Here's how the part is built. I have some questions about the finished solid (model axes, mm). Round coordinates to 2 decimals unless told otherwise and drop trailing zeros. Write each loop counter-clockwise with the first axis right and the second up, starting at its lowest first coordinate (ties: lowest second). Pieces come first, ordered by that corner, then holes. Notation, with made-up numbers: (-35.75, 78) -> (18.25, 78) arc R21 cw to (18.25, 82) -> close; hole circle Ø4 at (58, 29). An arc over 180 degrees is marked (long way). Put each result on its own line as item: value. Start each with the question number.
1. Suppose I cut it at A-A (y = 254). Please give me the cut outline in (x, z), then the cut area to 3 significant figures.
2. Suppose I cut it at B-B (x = 252.5). Please give me the cut outline in (y, z).
3. For pin 1 (5 mm diameter, centred on x = 248.5, z = 455.5, fed in from +Y); pin 2 (6 mm diameter, centred on x = 257.5, z = 166, fed in from -Y); pin 3 (6 mm diameter, centred on x = 249.5, y = 106, fed in from -Z), each with a flat end and sliding along its axis, tell me the tip position at first contact or that it passes through.
4. I need wall thicknesses on probe 1 along Z at (x, y) = (253.5, 222.5); probe 2 along Y at (x, z) = (253.5, 226). Which ranges of each line are inside material? Lowest first, please. Write a range as from..to.
5. Suppose I cut it at C-C (z = 377.5). Please give me the cut outline in (x, y).
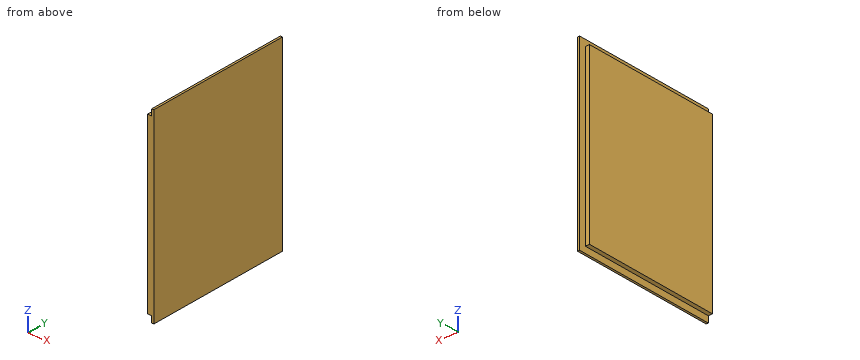
```python
from build123d import *

# Parameters (mm, degrees)
SKETCH056_W             = 410
SKETCH056_H             = 530
PAD021_DEPTH            = 18
SKETCH057_W             = 410
SKETCH057_H             = 18
POCKET034_DEPTH         = 12
SKETCH058_W             = 18
SKETCH058_H             = 530
POCKET035_DEPTH         = 12
BODY020_ROLL_ANGLE      = 90
BODY020_PLACEMENT_ANGLE = -90


with BuildPart() as part:
    # Sketch056 → Pad021 (new body)
    with BuildSketch(Plane.XY):
        with Locations((0, 265)):
            Rectangle(SKETCH056_W, SKETCH056_H)
    extrude(amount=PAD021_DEPTH)

    # Sketch057 (on Face6 of Pad021) → Pocket034 (cut)
    with BuildSketch(Plane.XY.offset(18)):
        with Locations((0, 9)):
            Rectangle(SKETCH057_W, SKETCH057_H)
        with Locations((0, 521)):
            Rectangle(SKETCH057_W, SKETCH057_H)
    extrude(amount=-POCKET034_DEPTH, mode=Mode.SUBTRACT)

    # Sketch058 (on Face9 of Pocket034) → Pocket035 (cut)
    with BuildSketch(Plane.XY.offset(18)):
        with Locations((-196, 265)):
            Rectangle(SKETCH058_W, SKETCH058_H)
    extrude(amount=-POCKET035_DEPTH, mode=Mode.SUBTRACT)


with BuildPart() as part_1:
    # Body020 roll: moved
    add(part.part.rotate(Axis((0, 0, 0), (1, 0, 0)), BODY020_ROLL_ANGLE))


with BuildPart() as part_2:
    # Body020 placement: moved
    add(part_1.part.moved(Location((263, 205, 0))).rotate(Axis((263, 205, 0), (0, 0, 1)), BODY020_PLACEMENT_ANGLE))


solid = part_2.part
```
Verdict:
1. outline: (245, 18) -> (257, 18) -> (257, 0) -> (263, 0) -> (263, 530) -> (257, 530) -> (257, 512) -> (245, 512) -> close
1. area: 9,110 mm^2
2. outline: (0, 18) -> (392, 18) -> (392, 512) -> (0, 512) -> close
3. pin 1: stops at y = 392
3. pin 2: stops at y = 0
3. pin 3: stops at z = 18
4. probe 1: z = 18..512
4. probe 2: y = 0..392
5. outline: (245, 0) -> (263, 0) -> (263, 410) -> (257, 410) -> (257, 392) -> (245, 392) -> close
